Answer from the drawing. Dimensions are ordinates in mm from the lowest x, y and z of the part. Give positions to 0.01 mm unless a question says otherwise; leave off trailing zeros. Write each loop counter-clockwise with the first axis right and the second up, starting at its lowest first coordinate (ties: lowest second). Pieces come first, ordered by that corner, then holes.
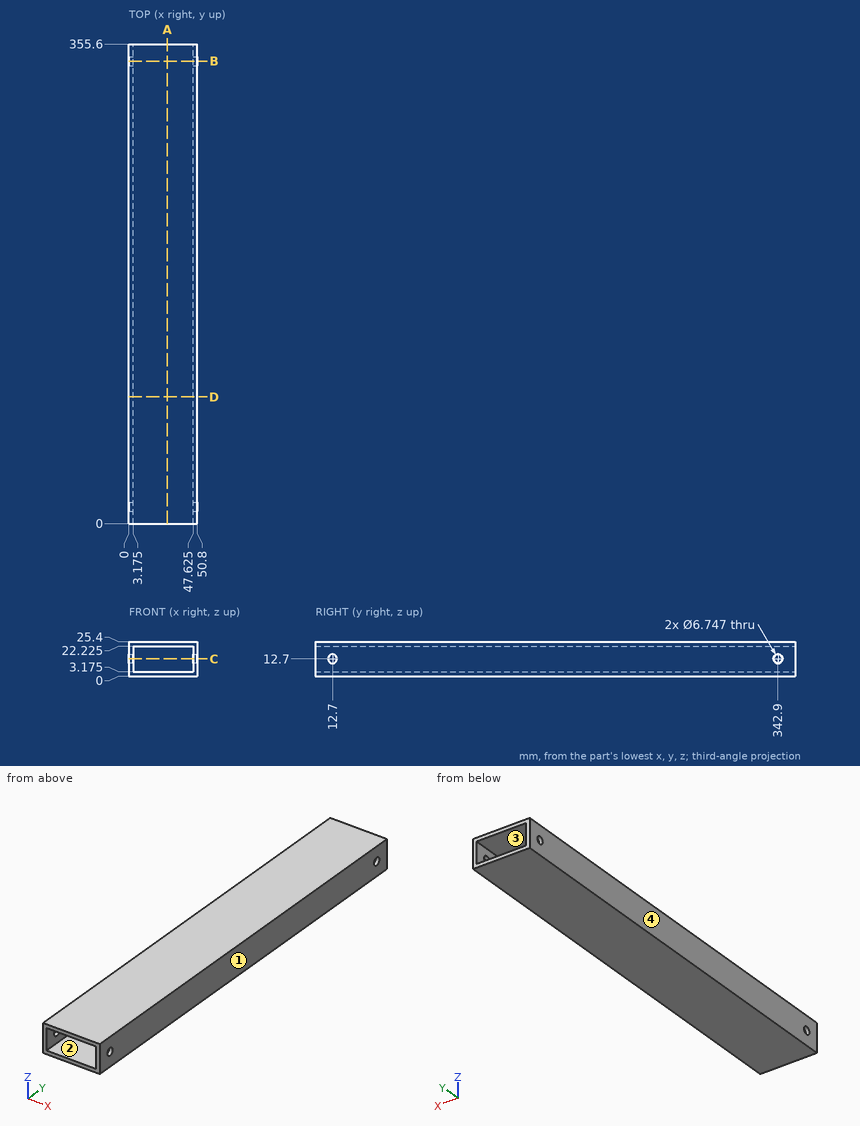
Item 1: This flat-tipped pin is pushed along its axis until it touches: pin 1 Ø1 at (x, z) = (26, 4) entering from -Y. Where does it stop, or does it pass through?
Result set:
pin 1: passes through
Item 2: Determine the mould class of the marked faces 1, 2, 3 and 4 for opening direction X: pulls with the +X half, pulls with the -X half, needs draft (parallel to the pull), parting line crosses it, or undercut.
Result set:
face 1: pulls with the +X half
face 2: undercut
face 3: undercut
face 4: pulls with the -X half
Item 3: Section A-A (x = 28.5) is taken. Write down the section's boundary in (y, z) (3 decimals), and give its area (3 significant figures).
Result set:
outline: (0, 0) - (355.6, 0) - (355.6, 3.175) - (0, 3.175) - close; (0, 22.225) - (355.6, 22.225) - (355.6, 25.4) - (0, 25.4) - close
area: 2,260 mm2
Item 4: Section D-D (y = 94) is taken. Write down the section's boundary in (x, z) (3 decimals).
Result set:
outline: (0, 0) - (50.8, 0) - (50.8, 25.4) - (0, 25.4) - close; hole (3.175, 3.175) - (47.625, 3.175) - (47.625, 22.225) - (3.175, 22.225) - close
Item 5: Section B-B (y = 342.9) is taken. Write down the section's boundary in (x, z) (1 decimal).
Result set:
outline: (0, 0) - (50.8, 0) - (50.8, 9.3) - (47.6, 9.3) - (47.6, 3.2) - (3.2, 3.2) - (3.2, 9.3) - (0, 9.3) - close; (0, 16.1) - (3.2, 16.1) - (3.2, 22.2) - (47.6, 22.2) - (47.6, 16.1) - (50.8, 16.1) - (50.8, 25.4) - (0, 25.4) - close
Item 6: Find the intervals of material crossed by line 1 along Y through (x, z) = (2.4, 12.7); line 2 along X through (y, z) = (182.5, 22) (3 decimals); line 3 along Z through (x, y) = (29, 93.5) (3 decimals), in increasing order.
Result set:
line 1: y = 0 to 9.33, 16.07 to 339.53, 346.27 to 355.6
line 2: x = 0 to 3.175, 47.625 to 50.8
line 3: z = 0 to 3.175, 22.225 to 25.4
Item 7: Section C-C (z = 12.7) is taken. Write down the section's boundary in (x, y) (1 decimal), and give its area (3 significant figures).
Result set:
outline: (0, 0) - (3.2, 0) - (3.2, 9.3) - (0, 9.3) - close; (0, 16.1) - (3.2, 16.1) - (3.2, 339.5) - (0, 339.5) - close; (0, 346.3) - (3.2, 346.3) - (3.2, 355.6) - (0, 355.6) - close; (47.6, 0) - (50.8, 0) - (50.8, 9.3) - (47.6, 9.3) - close; (47.6, 16.1) - (50.8, 16.1) - (50.8, 339.5) - (47.6, 339.5) - close; (47.6, 346.3) - (50.8, 346.3) - (50.8, 355.6) - (47.6, 355.6) - close
area: 2,170 mm2
